Autodesk Inventor part; units mm, degrees
ref_plane "YZ Plane" through (0, 0, 0) normal (1, 0, 0) x (0, 1, 0)
ref_plane "XZ Plane" through (0, 0, 0) normal (0, 1, 0) x (-1, 0, 0)
ref_plane "XY Plane" through (0, 0, 0) normal (0, 0, 1) x (1, 0, 0)
sketch "Sketch1" plane through (0, 0, 0) normal (0, 1, 0) x (-1, 0, 0)
  line L0 (-7, 41.5) -> (7, 41.5)
  line L1 (7, 41.5) -> (7, -41.5)
  line L2 (7, -41.5) -> (-7, -41.5)
  line L3 (-7, -41.5) -> (-7, 41.5)
  line L4 (-7, 41.5) -> (7, -41.5) construction
  line L5 (7, 41.5) -> (-7, -41.5) construction
  circle A0 centre (0, 34.5) radius 3.6
  circle A1 centre (0, -34.5) radius 3.6
  line L6 (13.7936, 0) -> (-15.5073, 0) construction
  point P0 (0, 0)
  dimension "d0" = 7.2
  dimension "d1" = 69
  dimension "d2" = 83
  dimension "d3" = 14
extrude "Extrusion1" add sketch "Sketch1" along normal mid plane 6
sketch "Sketch2" plane through (0, 0, 0) normal (1, 0, 0) x (0, 1, 0)
  circle A0 centre (9, 0) radius 3.5
  line L0 (10.1971, -3.2889) -> (3, -5.9084)
  line L1 (3, -41.5) -> (3, 41.5)
  line L2 (10.1971, 3.2889) -> (3, 5.9084)
  line L3 (9, 0) -> (-7.9221, 0) construction
  circle A1 centre (9, 0) radius 1.5
  point P0 (0, 0)
  point P1 (16.3025, 1.2439)
  point P2 (5, 7.6173)
  point P3 (5, -5.09)
  point P4 (3, 0)
  dimension "d6" = 7
  dimension "d11" = 20
  dimension "d12" = 6
  dimension "d13" = 3
extrude "Extrusion2" add sketch "Sketch2" along normal mid plane 2.4
fillet "Fillet1" radius 7 4 edges at (-7, 0, 41.5) (7, 0, 41.5) (-7, 0, -41.5) (7, 0, -41.5)
sketch "Sketch5" plane through (0, -3, 0) normal (0, -1, 0) x (1, 0, 0)
  arc A0 (-7, -34.5) -> (7, -34.5) centre (0, -34.5) ccw
  arc A1 (-7, -34.5) -> (7, -34.5) centre (0, -34.5) ccw
  line L0 (7, -34.5) -> (7, 34.5)
  arc A2 (7, 34.5) -> (-7, 34.5) centre (0, 34.5) ccw
  line L1 (-7, 34.5) -> (-7, -34.5)
  circle A3 centre (0, 34.5) radius 3.6
  circle A4 centre (0, -34.5) radius 3.6
  arc A5 (-5.5, -34.5) -> (5.5, -34.5) centre (0, -34.5) ccw
  line L2 (5.5, -34.5) -> (5.5, 34.5)
  arc A6 (5.5, 34.5) -> (-5.5, 34.5) centre (0, 34.5) ccw
  line L3 (-5.5, 34.5) -> (-5.5, -34.5)
  point P0 (0, 0)
  dimension "d32" = 1.5
extrude "Extrusion5" cut sketch "Sketch5" against normal blind 3 contours L3 A6 L2 A5
sketch "Sketch7" plane through (0, 0, 0) normal (0, 0, 1) x (1, 0, 0)
  point P0 (0, 0)
sketch "Sketch8" plane through (0, 0, 0) normal (0, 0, 1) x (1, 0, 0)
  line L0 (-5.5, -2.5) -> (-6.5, -1.5)
  line L1 (-6.5, -1.5) -> (-5.5, -0.5)
  line L2 (-6.5, -1.5) -> (-5.5, -1.5) construction
  line L3 (-5.5, -3) -> (-5.5, 0)
  point P0 (0, 0)
  dimension "d38" = 1
  dimension "d39" = 45
  dimension "d42" = 0.5
sketch3d "3D Sketch1"
  arc A0 (5.5, -3, -34.5) -> (3.8891, -3, -38.3891) centre (0, -3, -34.5) ccw
  arc A1 (3.8891, -3, -38.3891) -> (0, -3, -40) centre (0, -3, -34.5) ccw
  arc A2 (0, -3, -40) -> (-3.8891, -3, -38.3891) centre (0, -3, -34.5) ccw
  arc A3 (-3.8891, -3, -38.3891) -> (-5.5, -3, -34.5) centre (0, -3, -34.5) ccw
  line L0 (5.5, -3, -34.5) -> (5.5, -3, 34.5)
  arc A4 (-5.5, -3, 34.5) -> (-3.8891, -3, 38.3891) centre (0, -3, 34.5) ccw
  arc A5 (-3.8891, -3, 38.3891) -> (0, -3, 40) centre (0, -3, 34.5) ccw
  arc A6 (0, -3, 40) -> (3.8891, -3, 38.3891) centre (0, -3, 34.5) ccw
  arc A7 (3.8891, -3, 38.3891) -> (5.5, -3, 34.5) centre (0, -3, 34.5) ccw
  line L1 (-5.5, -3, 34.5) -> (-5.5, -3, -34.5)
sweep "Sweep1" cut profiles "Sketch8" path "3D Sketch1"
equation "\"d10\" = 0.5 * d3"
properties part number "Gripper_arms"
Can you work these out from the model? Positions are in its coordinate system, mm. A direction names the side the tool comes from. Give positions to 0.01 mm unless a question says otherwise; leave off trailing zeros. Loops run counter-clockwise (first coordinate to the right, second up) from the corner with the lowest first, then second, coordinate; pieces in that order, holes last. Notation, with made-up numbers: M 63,50.25 L 102,50.25 A20 ccw 102,79.25 Z; hole C 88,44.5 d6. An arc over 180 degrees is marked long. Use one line per item in the form item = value. Start each with the question number.
(1) I'm going to push flat-ended pins straight in: P1, Ø1, axis at x = 2, z = -12.5, coming from the -Y side; P2, Ø6, axis at x = 4, y = 1.5, coming from the -Z side; P3, Ø1, axis at x = 3, z = -18.5, coming from the +Y side. Where does each tip first touch, or does it pass through?
(2) Thinking about a two-plate mould opening in Z: for faces 6 (the flat face through (-1.2, 7, 0)), 7 (the flat face through (0, 6.6, 4.6)), 8 (the cylindrical face through (0.1, -0.3, 40)), 9 (the conical face through (5.46, -2.1, -36.73)), which applies, released by +Z, released by -Z, zero draft, split by the parting line, or undercut?
(3) Please list where these lines run through material, in increasing order: line 1 (Z direction, x = 0, y = 2.1); line 2 (X direction, y = 0.8, z = 34.5); line 3 (Z direction, x = 2.5, y = 2.5).
(4) I want a section at C-C, the plane z = -29. Write out the boundary of the cut face in (x, y), and give its area (3 significant figures).
(5) On a 3-axis mill with a long thin cutter (end or side, diameter ignored), from which of +Z, -Z, +X, -X, +Y, -Y can I reach the whole of each face in a straight line? I mean faces 1 (the conical face through (-5.435, -0.896, 36.786)), 2 (the flat face through (1.2, 7, 0)), 3 (the flat face through (0, 0, 1)), 4 (the cylindrical face through (0, 7.8, 0.9)), 5 (the cylindrical face through (0.47, 1.48, 30.93)). Say none if no direction works.
(6) I want a section at D-D, the plane y = 2. State how many separate pieces and enclosed holes the cut face has, and give its area (3 significant figures).
(7) I want a section at A-A, the plane z = 0. Write out the boundary of the cut face in (x, y), and give its area (3 significant figures).
(8) I want a section at B-B, the plane y = 9. Write out the boundary of the cut face in (x, z), and give its area (3 significant figures).
Worked out:
q1.P1 = 0
q1.P2 = -41.43
q1.P3 = 3
q2.face_6 = zero draft
q2.face_7 = released by +Z
q2.face_8 = undercut
q2.face_9 = undercut
q3.line_1 = -41.5 to -38.1, -30.9 to 30.9, 38.1 to 41.5
q3.line_2 = -7 to -3.6, 3.6 to 7
q3.line_3 = -41.04 to -37.09, -31.91 to 31.91, 37.09 to 41.04
q4.outline = M -7,-3 L -5.5,-3 L -5.5,-2.5 L -6.5,-1.5 L -5.5,-0.5 L -5.5,0 L 5.5,0 L 5.5,-0.5 L 6.5,-1.5 L 5.5,-2.5 L 5.5,-3 L 7,-3 L 7,3 L -7,3 Z
q4.area = 49.0 mm²
q5.face_1 = none
q5.face_2 = +Z, -Z, +X, +Y
q5.face_3 = -Y
q5.face_4 = +X, -X
q5.face_5 = +Y, -Y
q6.separate_pieces = 1
q6.enclosed_holes = 2
q6.area = 1,040 mm²
q7.outline = M -7,-3 L -5.5,-3 L -5.5,-2.5 L -6.5,-1.5 L -5.5,-0.5 L -5.5,0 L 5.5,0 L 5.5,-0.5 L 6.5,-1.5 L 5.5,-2.5 L 5.5,-3 L 7,-3 L 7,3 L 1.2,3 L 1.2,7.5 L -1.2,7.5 L -1.2,3 L -7,3 Z; M -1.2,10.5 L 1.2,10.5 L 1.2,12.5 L -1.2,12.5 Z
q7.area = 64.6 mm²
q8.outline = M -1.2,-3.72 L 1.2,-3.72 L 1.2,-1.5 L -1.2,-1.5 Z; M -1.2,1.5 L 1.2,1.5 L 1.2,3.72 L -1.2,3.72 Z
q8.area = 10.7 mm²
